Source: CAD feature listing. Evaluate the final solid. Frame: model axes, mm. A direction names the side the tool comes from. Give positions to 0.01 mm unless a question says otherwise; leave off trailing zeros. Loops run counter-clockwise (first coordinate to the right, second up) from the corner with the lowest first, then second, coordinate; pieces in that order, holes last. Notation, with made-up numbers: M 48,-26 L 79,-26 A19 ccw 79,-5 Z; hole C 41,54 d1. An arc over 180 degrees is marked long. Answer in a Markdown table with one row per item.
```python
from build123d import *

# Parameters (mm, degrees)
F0_W     = 35
F0_H     = 10.25
F0_W_2   = 10.25
F0_H_2   = 25
F1_DEPTH = 10


with BuildPart() as f1:
    # F0 (on Top) → F1 (new body)
    with BuildSketch(Plane.XY):
        with BuildLine():
            Line((140, 110), (-140, 110))
            ThreePointArc((-140, 110), (-147.071068, 107.071068), (-150, 100))
            Line((-150, 100), (-150, -100))
            ThreePointArc((-150, -100), (-147.071068, -107.071068), (-140, -110))
            Line((-140, -110), (140, -110))
            ThreePointArc((140, -110), (147.071068, -107.071068), (150, -100))
            Line((150, -100), (150, 100))
            ThreePointArc((150, 100), (147.071068, 107.071068), (140, 110))
        make_face()
        Polygon((-105.125, -100.125), (-140.125, -100.125), (-140.125, -75.125), (-129.875, -75.125), (-129.875, -89.878049), (-105.125, -89.875), align=None, mode=Mode.SUBTRACT)
        with Locations((-52.625, -95)):
            Rectangle(F0_W, F0_H, mode=Mode.SUBTRACT)
        with Locations((-135, -37.625)):
            Rectangle(F0_W_2, F0_H_2, mode=Mode.SUBTRACT)
        with Locations((52.625, -95)):
            Rectangle(F0_W, F0_H, mode=Mode.SUBTRACT)
        Polygon((129.875, -75.125), (140.125, -75.125), (140.125, -100.125), (105.125, -100.125), (105.125, -89.875), (129.875, -89.878049), align=None, mode=Mode.SUBTRACT)
        with Locations((135, -37.625)):
            Rectangle(F0_W_2, F0_H_2, mode=Mode.SUBTRACT)
        with Locations((-135, 37.625)):
            Rectangle(F0_W_2, F0_H_2, mode=Mode.SUBTRACT)
        Polygon((-129.875, 75.125), (-140.125, 75.125), (-140.125, 100.125), (-105.125, 100.125), (-105.125, 89.875), (-129.875, 89.878049), align=None, mode=Mode.SUBTRACT)
        with Locations((-52.625, 95)):
            Rectangle(F0_W, F0_H, mode=Mode.SUBTRACT)
        with Locations((135, 37.625)):
            Rectangle(F0_W_2, F0_H_2, mode=Mode.SUBTRACT)
        with Locations((52.625, 95)):
            Rectangle(F0_W, F0_H, mode=Mode.SUBTRACT)
        Polygon((105.125, 89.875), (105.125, 100.125), (140.125, 100.125), (140.125, 75.125), (129.875, 75.125), (129.875, 89.878049), align=None, mode=Mode.SUBTRACT)
    extrude(amount=F1_DEPTH)


solid = f1.part
```
Q1. Section query A-A (y = 32.5). Output: boundary loops of the cut face in (x, z) (3 decimals), plus the area to 4 significant figures.
Values follow:
| item | result |
|---|---|
| outline | M -150,0 L -140.125,0 L -140.125,10 L -150,10 Z; M -129.875,0 L 129.875,0 L 129.875,10 L -129.875,10 Z; M 140.125,0 L 150,0 L 150,10 L 140.125,10 Z |
| area | 2,795 mm^2 |
Q2. Section query B-B (x = 59). Output: boundary loops of the cut face in (y, z) (3 decimals).
Values follow:
| item | result |
|---|---|
| outline | M -110,0 L -100.125,0 L -100.125,10 L -110,10 Z; M -89.875,0 L 89.875,0 L 89.875,10 L -89.875,10 Z; M 100.125,0 L 110,0 L 110,10 L 100.125,10 Z |
Q3. Ray query, probe 1 along X at (y, z) = (-50, 9.5) (3 decimals); probe 2 along Y at (x, z) = (108.5, 1.75) (3 decimals); probe 3 along X at (y, z) = (-94.5, 3) (3 decimals). Return the intervals inside material, ascending. Write a range as from..to.
Values follow:
| item | result |
|---|---|
| probe 1 | -150..-140.125, -129.875..129.875, 140.125..150 |
| probe 2 | -110..-100.125, -89.875..89.875, 100.125..110 |
| probe 3 | -150..-140.125, -105.125..-70.125, -35.125..35.125, 70.125..105.125, 140.125..150 |
Q4. Reachability of faces 1 (the flat face through (-2, 2, 10)), 2 (the flat face through (-140.125, -88, 5)) from +Z, -Z, +X, -X, +Y, -Y: full face, straight path, thin tool, end or side. Return the list, or none.
Values follow:
| item | result |
|---|---|
| face 1 | +Z, +X, -X, +Y, -Y |
| face 2 | +Z, -Z |
Q5. Section query C-C (z = 2.25). Give the number of separate pieces and of enclosed holes in the cut face, plus the area to 3 significant figures.
Values follow:
| item | result |
|---|---|
| separate pieces | 1 |
| enclosed holes | 12 |
| area | 61,400 mm^2 |
